Model file for the job. Use its own axes, mm. Face numbers are marked on the shaded views. Round coordinates to 2 decimals unless told otherwise and drop trailing zeros. Order: outer loops, then holes, each group sorted by start corner. A loop starts at its lowest first (then second) coordinate and runs counter-clockwise, first axis right, second up. Notation, with made-up numbers: (-38.75, 36.5) - (-0.75, 36.5) arc R15 ccw to (-0.75, 42.5) - close; hole circle Ø2 at (41.5, 58). An arc over 180 degrees is marked (long way). Answer as CSV lines item,"result". Start each with the question number.
1. Band-saw the part on A-A on y = 27.94. List the corners of the cut face in (x, z), then the cut area to 3 significant figures.
2. Pull direction Z, two halves, no side cores. Call the marked faces 1, 2, 3 and 4: released by +Z, released by -Z, zero draft, split by the parting line, or undercut.
3. Band-saw the part on C-C on x = 19.5. List the corners of the cut face in (y, z).
4. Band-saw the part on D-D on y = 50. List the corners of the cut face in (x, z).
5. Pin check, flat tips, straight feed: pin 1 Ø2 at (y, z) = (44.45, -6.985) entering from +X; pin 2 Ø1.5 at (y, z) = (28, -14.5) entering from +X; pin 3 Ø7 at (x, y) = (14.5, 30) entering from +Z; pin 4 Ø3.5 at (x, y) = (17, 5) entering from +Z. Stop position of each tip, or through.
6. Wall check: line 1 along Y through (x, z) = (1.05, 1.27); line 2 along Y through (x, z) = (1.1, -15.24); line 3 along X through (y, z) = (15, -27). Give the ranges that are in metal, low to high. Write a range as [from, to].
7. Band-saw the part on B-B on z = -15.24. List the corners of the cut face in (x, y), then the cut area to 3 significant figures.
```python
from build123d import *

# Parameters (mm, degrees)
SKETCH1_W             = 30.48
SKETCH1_H             = 57.15
BOSS_EXTRUDE1_DEPTH   = 1.524
SKETCH2_W             = 1.524
SKETCH2_H             = 57.15
SKETCH2_H_2           = 7.62
BOSS_EXTRUDE2_DEPTH   = 22.86
SKETCH3_W             = 1.524
SKETCH3_H             = 45.72
BOSS_EXTRUDE3_DEPTH   = 5.08
F_2_CLEARANCE_HOLE1_D = 2.4384


with BuildPart() as part:
    # Sketch1 → Boss-Extrude1 (new body)
    with BuildSketch(Plane(origin=(0, 0, 0), x_dir=(0, 0, -1), z_dir=(1, 0, 0))):
        with Locations((15.24, 28.575)):
            Rectangle(SKETCH1_W, SKETCH1_H)
    extrude(amount=BOSS_EXTRUDE1_DEPTH)

    # Sketch2 → Boss-Extrude2 (add)
    with BuildSketch(Plane(origin=(1.524, 0, 0), x_dir=(0, 0, -1), z_dir=(1, 0, 0))):
        with Locations((29.718, 28.575)):
            Rectangle(SKETCH2_W, SKETCH2_H)
        with Locations((0.762, 3.81)):
            Rectangle(SKETCH2_W, SKETCH2_H_2)
    extrude(amount=BOSS_EXTRUDE2_DEPTH)

    # Sketch3 → Boss-Extrude3 (add)
    with BuildSketch(Plane.XY):
        with Locations((0.762, 34.29)):
            Rectangle(SKETCH3_W, SKETCH3_H)
    extrude(amount=BOSS_EXTRUDE3_DEPTH)

    # #2 Clearance Hole1 (through all)
    with Locations(Plane(origin=(1.524, 0, 0), x_dir=(0, 0, -1), z_dir=(1, 0, 0))):
        with Locations((-1.27, 36.195), (15.24, 36.195), (6.985, 44.45), (6.985, 27.94), (6.985, 11.43), (15.24, 19.685), (-1.27, 19.685)):
            Hole(F_2_CLEARANCE_HOLE1_D / 2)


solid = part.part
```
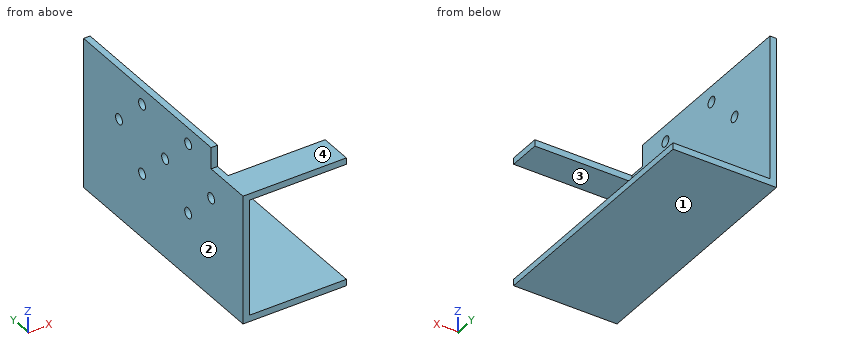
Reply:
1,outline,"(0, -30.48) - (24.38, -30.48) - (24.38, -28.96) - (1.52, -28.96) - (1.52, -8.2) - (0, -8.2) - close; (0, -5.77) - (1.52, -5.77) - (1.52, 5.08) - (0, 5.08) - close"
1,area,"85.3 mm2"
2,face 1,"released by -Z"
2,face 2,"zero draft"
2,face 3,"undercut"
2,face 4,"released by +Z"
3,outline,"(0, -30.48) - (57.15, -30.48) - (57.15, -28.96) - (0, -28.96) - close; (0, -1.52) - (7.62, -1.52) - (7.62, 0) - (0, 0) - close"
4,outline,"(0, -30.48) - (24.38, -30.48) - (24.38, -28.96) - (1.52, -28.96) - (1.52, 5.08) - (0, 5.08) - close"
5,pin 1,"passes through"
5,pin 2,"stops at x = 1.52"
5,pin 3,"stops at z = -28.96"
5,pin 4,"stops at z = 0"
6,line 1,"y = [11.43, 18.47], [20.9, 34.98], [37.41, 57.15]"
6,line 2,"y = [0, 18.47], [20.9, 34.98], [37.41, 57.15]"
6,line 3,"x = [0, 1.52]"
7,outline,"(0, 0) - (1.52, 0) - (1.52, 18.47) - (0, 18.47) - close; (0, 20.9) - (1.52, 20.9) - (1.52, 34.98) - (0, 34.98) - close; (0, 37.41) - (1.52, 37.41) - (1.52, 57.15) - (0, 57.15) - close"
7,area,"79.7 mm2"
